Check sheet for the modelled part. Datum: model origin and axes. Units: mm. A direction names the side the tool comes from. Coordinates: 2 decimals unless noted, no trailing zeros. Loops run counter-clockwise (first coordinate to the right, second up) from the corner with the lowest first, then second, coordinate; pieces in that order, holes last. Notation, with made-up numbers: (-36, 71) -> (-16, 71) arc R24 cw to (-16, 93) -> close; hole circle Ø3 at (46, -12). An arc over 180 degrees is marked (long way). Use one line per item in the form item = value.
from build123d import *

# Parameters (mm, degrees)
BOSS_EXTRUDE1_DEPTH = 2.54
BOSS_EXTRUDE2_REACH = 281.854
SKETCH3_R           = 9.525
CUT_EXTRUDE1_DEPTH  = 286.222196584
SKETCH4_R           = 6.35
CUT_EXTRUDE2_DEPTH  = 286.222196584
SKETCH5_W           = 166.701294092
SKETCH5_H           = 254.634379314
CUT_EXTRUDE3_DEPTH  = 25.4


with BuildPart() as part:
    # Sketch1 → Boss-Extrude1 (new body)
    with BuildSketch(Plane.XY):
        Polygon((-154.89754402, 192.409602109), (-154.89754402, -106.378927356), (-137.076300146, -113.087952221), (-112.691620976, -88.703273051), (0, -88.703273051), (24.38467917, -113.087952221), (48.30245598, -100.895612636), (48.30245598, -46.801532207), (48.30245598, 185.942762537), (28.636463872, 185.942762537), (28.636463872, 156.398467793), (-137.076300146, 156.398467793), (-137.076300146, 192.409602109), align=None)
    extrude(amount=BOSS_EXTRUDE1_DEPTH)

    # Boss-Extrude2: up to this face of the body (flat: up to its plane)
    boss_extrude2_end = Plane(part.part.faces().sort_by_distance((-154.89754402, 43.015337376, 1.27))[0])
    # Sketch2 → Boss-Extrude2 (add, up to the picked face)
    with BuildSketch(Plane(origin=(48.30245598, 0, 0), x_dir=(0, 0, -1), z_dir=(1, 0, 0)), mode=Mode.PRIVATE) as boss_extrude2_sk1:
        Polygon((0, 170.234631614), (21.075391445, 191.310023059), (41.695088388, 191.310023059), (55.136253414, 145.191484573), (55.136253414, -7.208515427), (9.464727664, -72.14198279), (9.464727664, -49.306219915), (0, -39.841492251), align=None)
    boss_extrude2_tool1 = split(extrude(boss_extrude2_sk1.sketch, amount=-BOSS_EXTRUDE2_REACH, mode=Mode.PRIVATE), bisect_by=boss_extrude2_end, keep=Keep.BOTH, mode=Mode.PRIVATE)
    add(boss_extrude2_tool1.solids().sort_by(Axis((48.302456, 70.213482, -26.354357), (-1, 0, 0)))[0])

    # Sketch3 → Cut-Extrude1 (cut, through all)
    with BuildSketch(Plane(origin=(48.30245598, 0, 0), x_dir=(0, 0, -1), z_dir=(1, 0, 0))):
        with Locations((36.933690773, 143.349042369)):
            Circle(SKETCH3_R)
        with Locations((36.933690773, 0)):
            Circle(SKETCH3_R)
    extrude(amount=-CUT_EXTRUDE1_DEPTH, mode=Mode.SUBTRACT)

    # Sketch4 → Cut-Extrude2 (cut, through all)
    with BuildSketch(Plane(origin=(48.30245598, 0, 0), x_dir=(0, 0, -1), z_dir=(1, 0, 0))):
        with Locations((11.650142798, 161.721177387)):
            Circle(SKETCH4_R)
        with Locations((11.736614281, 9.321201919)):
            Circle(SKETCH4_R)
        with Locations((11.650142798, 125.160679587)):
            Circle(SKETCH4_R)
        with Locations((11.650142798, 91.064352978)):
            Circle(SKETCH4_R)
        with Locations((11.650142798, 51.543610773)):
            Circle(SKETCH4_R)
        with Locations((11.736614281, -30.597539694)):
            Circle(SKETCH4_R)
    extrude(amount=-CUT_EXTRUDE2_DEPTH, mode=Mode.SUBTRACT)

    # Sketch5 → Cut-Extrude3 (cut)
    with BuildSketch(Plane.XY.offset(2.54)):
        with Locations((-44.614217323, 53.073750236)):
            Rectangle(SKETCH5_W, SKETCH5_H)
    extrude(amount=-CUT_EXTRUDE3_DEPTH, mode=Mode.SUBTRACT)


solid = part.part
(1) Section check C-C, the plane x = 15. Record the boundary of the cut face in (y, z) (3 decimals).
Established:
outline = (-103.703, 0) -> (-74.243, 0) -> (-74.243, 2.54) -> (-103.703, 2.54) -> close; (-53.097, -22.86) -> (-7.209, -55.136) -> (145.191, -55.136) -> (191.31, -41.695) -> (191.31, -21.075) -> (180.391, -10.156) -> (180.391, -22.86) -> close; hole circle Ø19.05 at (0, -36.934); hole circle Ø19.05 at (143.349, -36.934)
(2) Section check A-A, the plane x = -53. Record the boundary of the cut face in (y, z) (3 decimals), plus the area to 3 significant figures.
Established:
outline = (-88.703, 0) -> (-74.243, 0) -> (-74.243, 2.54) -> (-88.703, 2.54) -> close; (-53.097, -22.86) -> (-7.209, -55.136) -> (145.191, -55.136) -> (191.31, -41.695) -> (191.31, -21.075) -> (180.391, -10.156) -> (180.391, -22.86) -> close; hole circle Ø19.05 at (0, -36.934); hole circle Ø19.05 at (143.349, -36.934)
area = 6,380 mm²
(3) Mould release check, pull along Y, two halves, no side actions. Record for faces 3 (the flat face through (-52, 191.31, -31)), 4 (the flat face through (-51.9, -32, -37.7)), 5 (the flat face through (-141, -61, -9.465)), 6 (the cylindrical face through (43.586, 155.522, -10.274)): +Y half, -Y half, draft (parallel to the pull), parting line (faces both ways), or undercut.
Established:
face_3 = +Y half
face_4 = -Y half
face_5 = draft
face_6 = undercut
(4) Tool access check on faces 1 (the flat face through (-146.112, -109.686, 1.252)), 2 (the flat face through (38.736, 51, -4)). Record the directions out of +Z, -Z, +X, -X, +Y, -Y that give a thin tool (end or side, any length) a straight path to the whole face; none if there is none.
Established:
face_1 = +Z, -Z, -X, -Y
face_2 = +Z
(5) Scan lines: line 1 along X through (y, z) = (55, -2); line 2 along Y through (x, z) = (-104, -31); line 3 along Y through (x, z) = (-13, -34.5). Record each from-to range of solid material in increasing order.
Established:
line_1 = -154.9 to -127.96, 38.74 to 48.3
line_2 = -41.52 to -7.45, 7.45 to 135.9, 150.8 to 191.31
line_3 = -36.55 to -9.21, 9.21 to 134.14, 152.56 to 191.31
(6) Section check B-B, the plane z = -37. Record the boundary of the cut face in (x, y), plus the area to 3 significant figures.
Established:
outline = (-154.9, -32.99) -> (48.3, -32.99) -> (48.3, -9.52) -> (-154.9, -9.52) -> close; (-154.9, 9.52) -> (48.3, 9.52) -> (48.3, 133.82) -> (-154.9, 133.82) -> close; (-154.9, 152.87) -> (48.3, 152.87) -> (48.3, 191.31) -> (-154.9, 191.31) -> close
area = 37,800 mm²
(7) Go/stop test with flat-tipped pins: P1, Ø12, axis at x = -104.5, y = 161.5, coming from the -Z side; P2, Ø5, axis at x = 6.5, z = -18, coming from the +Y side; P3, Ø4, axis at x = -60, z = -34, coming from the -Y side; P4, Ø6, axis at x = -120, z = -5, coming from the +Y side. Record where each tip stops, or that it passes through.
Established:
P1 = -52.13
P2 = 190.73
P3 = -40.1
P4 = through
